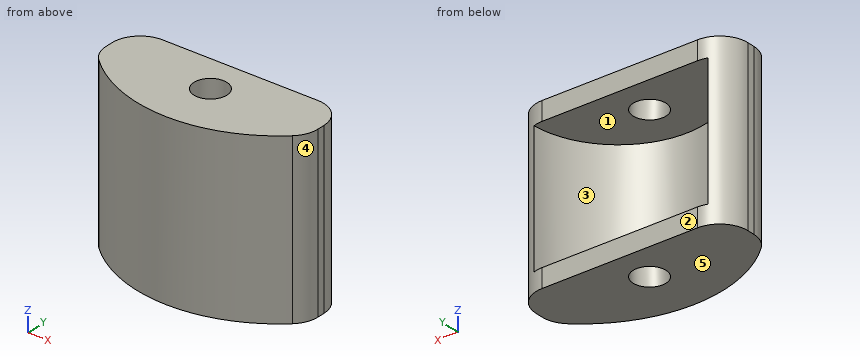
```python
from build123d import *

# Parameters (mm, degrees)
SKETCH1_W               = 22.5
SKETCH1_H               = 18
BOSS_EXTRUDE1_DEPTH     = 10
CUT_EXTRUDE1_DEPTH      = 24.464068275
CUT_EXTRUDE1_DEPTH_BACK = 24.464068275
SKETCH2_R               = 1.75
CUT_EXTRUDE2_DEPTH      = 14
CUT_EXTRUDE3_REACH      = 19.532
SKETCH4_W               = 11.529065942
SKETCH4_H               = 14
FILLET1_R               = 3


with BuildPart() as part:
    # Sketch1 → Boss-Extrude1 (new body)
    with BuildSketch(Plane(origin=(0, 0, 0), x_dir=(1, 0, 0), z_dir=(0, 1, 0))):
        Rectangle(SKETCH1_W, SKETCH1_H)
    extrude(amount=BOSS_EXTRUDE1_DEPTH)

    # Sketch2 → Cut-Extrude1 (cut, two sides: drawn at the far end of the back side and taken through both)
    with BuildSketch(Plane.XY.offset(9).offset(-CUT_EXTRUDE1_DEPTH_BACK)):
        with Locations((0, 6)):
            Circle(SKETCH2_R)
        with BuildLine():
            Line((-11.25, 5), (-11.25, 0))
            Line((-11.25, 0), (11.25, 0))
            Line((11.25, 0), (11.25, 5))
            ThreePointArc((11.25, 5), (0, 0.01), (-11.25, 5))
        make_face()
    extrude(amount=CUT_EXTRUDE1_DEPTH + CUT_EXTRUDE1_DEPTH_BACK, mode=Mode.SUBTRACT)

    # Sketch3 → Cut-Extrude2 (cut)
    with BuildSketch(Plane.XY.offset(7)):
        with BuildLine():
            ThreePointArc((-9.233945582, 9.952114837), (0, 0.969656164), (9.233945582, 9.952114837))
            ThreePointArc((9.233945582, 9.952114837), (7.547885163, 11.733945582), (5.766054418, 10.047885163))
            ThreePointArc((5.766054418, 10.047885163), (0, 4.438869486), (-5.766054418, 10.047885163))
            ThreePointArc((-5.766054418, 10.047885163), (-7.547885163, 11.733945582), (-9.233945582, 9.952114837))
        make_face()
    extrude(amount=-CUT_EXTRUDE2_DEPTH, mode=Mode.SUBTRACT)

    # Sketch4 → Cut-Extrude3 (cut, up to next)
    with BuildSketch(Plane(origin=(0, 10, 0), x_dir=(1, 0, 0), z_dir=(0, 1, 0)), mode=Mode.PRIVATE) as cut_extrude3_sk1:
        Rectangle(SKETCH4_W, SKETCH4_H)
    cut_extrude3_tool1 = extrude(cut_extrude3_sk1.sketch, amount=-CUT_EXTRUDE3_REACH, mode=Mode.PRIVATE) & part.part
    add(cut_extrude3_tool1.solids().sort_by_distance((0, 10, 0))[0], mode=Mode.SUBTRACT)

    # Fillet1
    # the kernel refuses this fillet: 3 mm, written as the material it takes off along each edge
    with BuildSketch(Plane(origin=(11.25, 5, 12.435069568), x_dir=(0, 1, 0), z_dir=(0, 0, -1))) as fillet1_piece_1:
        with BuildLine():
            CenterArc((1.230754269, -3), FILLET1_R, 90, 47.349204062)
            ThreePointArc((-0.975735859, -0.967415115), (-0.498821765, -0.472659508), (0, 0))
            Line((0, 0), (1.230754269, 0))
        make_face()
    extrude(amount=24.870139136, mode=Mode.SUBTRACT)
    with BuildSketch(Plane(origin=(-11.25, 5, 12.435069568), x_dir=(0, 1, 0), z_dir=(0, 0, -1))) as fillet1_piece_2:
        with BuildLine():
            CenterArc((1.230754269, 3), FILLET1_R, 222.650795938, 47.349204062)
            ThreePointArc((-0.975735859, 0.967415115), (-0.498821765, 0.472659508), (0, 0))
            Line((0, 0), (1.230754269, 0))
        make_face()
    extrude(amount=24.870139136, mode=Mode.SUBTRACT)
    with BuildSketch(Plane(origin=(11.25, 10, -16.5), x_dir=(-1, 0, 0), z_dir=(0, 0, 1))) as fillet1_piece_3:
        with BuildLine():
            CenterArc((FILLET1_R, FILLET1_R), FILLET1_R, 180, 90)
            Line((0, FILLET1_R), (0, 0))
            Line((0, 0), (FILLET1_R, 0))
        make_face()
    extrude(amount=33, mode=Mode.SUBTRACT)
    with BuildSketch(Plane(origin=(-11.25, 10, 16.5), x_dir=(0, -1, 0), z_dir=(0, 0, -1))) as fillet1_piece_4:
        with BuildLine():
            CenterArc((FILLET1_R, -FILLET1_R), FILLET1_R, 90, 90)
            Line((0, -FILLET1_R), (0, 0))
            Line((0, 0), (FILLET1_R, 0))
        make_face()
    extrude(amount=33, mode=Mode.SUBTRACT)


solid = part.part
```
CAD build for the part. Positions are in the model's coordinates, mm. Face numbers are marked on the shaded views. A direction names the side the tool comes from. Coordinates: 2 decimals unless noted, no trailing zeros. Order: outer loops, then holes, each group sorted by start corner. A loop starts at its lowest first (then second) coordinate and runs counter-clockwise, first axis right, second up. Notation, with made-up numbers: (53.25, 53.5) - (102.25, 53.5) arc R24 cw to (102.25, 86.5) - close; hole circle Ø9 at (13, -25). An arc over 180 degrees is marked (long way). Answer in a Markdown table with one row per item.
1. Flat gauge pins, fed straight in: P1, Ø3, axis at x = 6.5, z = 0, coming from the -Y side; P2, Ø5, axis at x = 7, z = 3.5, coming from the -Y side. Where does each tip first touch, or does it go through?
Answer:
| item | result |
|---|---|
| P1 | y = 0.86 |
| P2 | y = 0.69 |
2. Drill centre lines: L1, parallel to Z at x = 2.5, y = 6.5; L2, parallel to X at y = 3, z = 0; L3, parallel to X at y = 6, z = -8.6. Where is each one in solid material? Low to high. Write a range as from..to.
Answer:
| item | result |
|---|---|
| L1 | -9..-7, 7..9 |
| L2 | -9.05..-5.78, 5.78..9.05 |
| L3 | -11.24..-1.75, 1.75..11.24 |
3. Slice it at A-A, the plane x = 0. List the corners of the cut face in (y, z).
Answer:
| item | result |
|---|---|
| outline | (0.01, -9) - (4.25, -9) - (4.25, -7) - (0.97, -7) - (0.97, 7) - (4.25, 7) - (4.25, 9) - (0.01, 9) - close; (7.75, -9) - (10, -9) - (10, -7) - (7.75, -7) - close; (7.75, 7) - (10, 7) - (10, 9) - (7.75, 9) - close |
4. Slice it at D-D, the plane x = -6.75. List the corners of the cut face in (y, z).
Answer:
| item | result |
|---|---|
| outline | (1.59, -9) - (10, -9) - (10, -7) - (3.9, -7) - (3.9, 7) - (10, 7) - (10, 9) - (1.59, 9) - close |
5. 3-axis set-ups, long thin cutter, end or side, ignore diameter. For the marked faces 1 and 2: which of +Z, -Z, +X, -X, +Y, -Y reach the whole face in a straight line?
Answer:
| item | result |
|---|---|
| face 1 | +Y |
| face 2 | +Z, -Z, +X, -X, +Y |
6. Pull direction Z, two halves, no side cores. Call the marked faces 3, 4 and 5: +Z half, -Z half, draft (parallel to the pull), parting line (faces both ways), or undercut.
Answer:
| item | result |
|---|---|
| face 3 | undercut |
| face 4 | draft |
| face 5 | -Z half |
7. Slice it at C-C, the plane y = 5. List the corners of the cut face in (x, z), then the cut area to 3 significant figures.
Answer:
| item | result |
|---|---|
| outline | (-10.99, -9) - (-1.44, -9) - (-1.44, -7) - (-7.63, -7) - (-7.63, 7) - (-1.44, 7) - (-1.44, 9) - (-10.99, 9) - close; (1.44, -9) - (10.99, -9) - (10.99, 9) - (1.44, 9) - (1.44, 7) - (7.63, 7) - (7.63, -7) - (1.44, -7) - close |
| area | 170 mm² |
